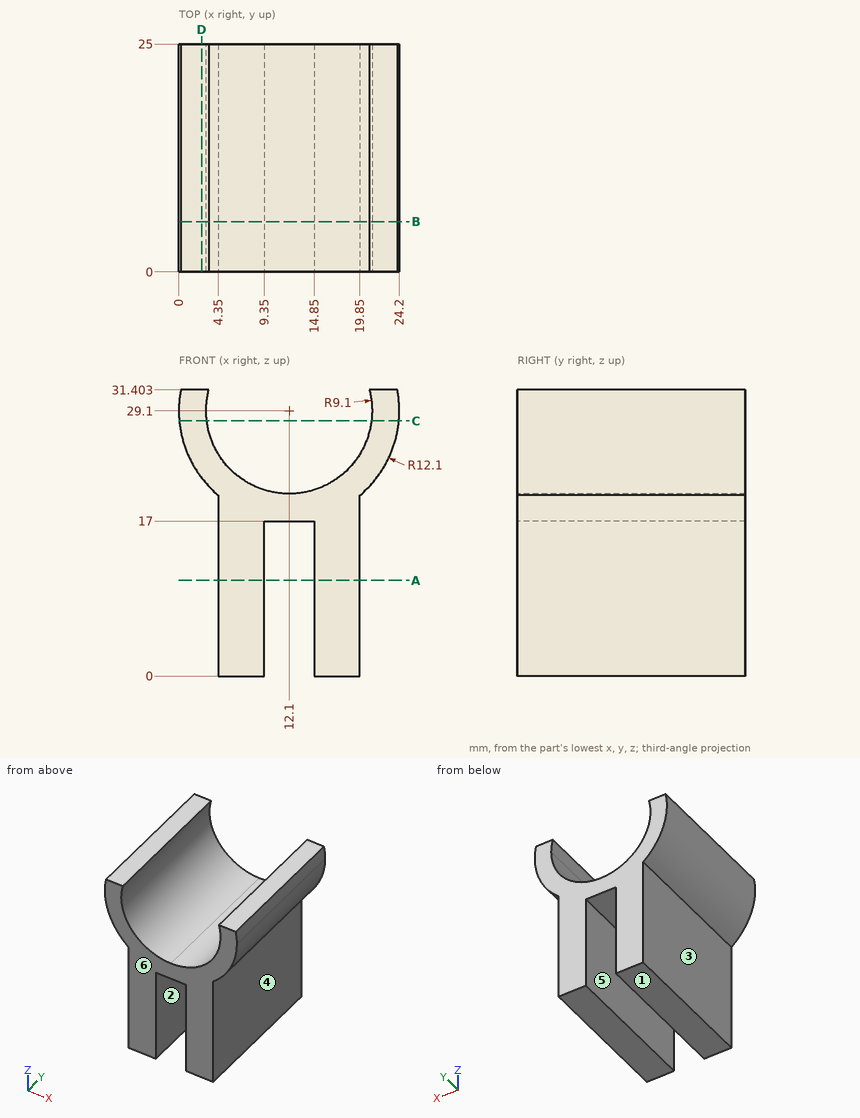
Answer from the drawing. Dimensions are ordinates in mm from the lowest x, y and z of the part. A direction names the side the tool comes from. Give positions to 0.01 mm unless a question says otherwise; leave off trailing zeros. Order: outer loops, then holes, each group sorted by start corner. A loop starts at its lowest first (then second) coordinate and runs counter-clockwise, first axis right, second up. Notation, with made-up numbers: (73.5, 29.25) - (131.5, 29.25) arc R21 cw to (131.5, 34.25) - close; hole circle Ø1 at (85.5, 7.25). An arc over 180 degrees is marked (long way). One line per item, written item: value. Start each with the question number.
1) Given pin 1 Ø3 at (x, y) = (12.5, 21.5) entering from -Z; pin 2 Ø12 at (y, z) = (6, 22.5) entering from -X (3 decimals); pin 3 Ø2 at (y, z) = (15, 20) entering from -X, each flat-ended and moving along its own axis, determine where each tip first touches the part or whether it passes through.
2) Find the intervals of material crossed by L1, parallel to X at y = 2.25, z = 6.5; L2, parallel to Z at x = 12, y = 15.25; L3, parallel to X at y = 21, z = 24, in increasing order.
3) The mould has two halves that part along X. Classify the marked faces 1, 2 and 3: released by +X, released by -X, zero draft, split by the parting line, or undercut.
4) A cutting plane is placed at C-C on z = 28. Give the vertices of the cut face in (x, y).
5) A cutting plane is placed at B-B on y = 5.5. Give the vertices of the cut face in (x, z), then the cut area to 3 significant figures.
6) A cutting plane is placed at D-D on x = 2.5. Give the vertices of the cut face in (y, z) (1 decimal), then the cut area to 3 significant figures.
7) A cutting plane is placed at A-A on z = 10.5. Give the vertices of the cut face in (x, y), then the cut area to 3 significant figures.
8) A tool of negligible diameter and unlimited length cuts with its end or side. For the marked faces 4, 5 and 6, from which of +Z, -Z, +X, -X, +Y, -Y can it reach the whole face along a straight path? Write none if from no direction.
Answer sheet:
1. pin 1: stops at z = 17
1. pin 2: stops at x = 0.015
1. pin 3: stops at x = 3.11
2. L1: x = 4.35 to 9.35, 14.85 to 19.85
2. L2: z = 17 to 20
2. L3: x = 1.13 to 4.56, 19.64 to 23.07
3. face 1: zero draft
3. face 2: undercut
3. face 3: released by -X
4. outline: (0.05, 0) - (3.07, 0) - (3.07, 25) - (0.05, 25) - close; (21.13, 0) - (24.15, 0) - (24.15, 25) - (21.13, 25) - close
5. outline: (0.22, 31.4) arc R12.1 ccw to (4.35, 19.81) - (4.35, 0) - (9.35, 0) - (9.35, 17) - (14.85, 17) - (14.85, 0) - (19.85, 0) - (19.85, 19.81) arc R12.1 ccw to (24.2, 29.1) arc R12.1 ccw to (23.98, 31.4) - (20.9, 31.4) arc R9.1 cw to (21.2, 29.1) arc R9.1 cw to (12.1, 20) arc R9.1 cw to (3.3, 31.4) - close
5. area: 298 mm2
6. outline: (0, 21.7) - (25, 21.7) - (25, 31.4) - (0, 31.4) - close
6. area: 242 mm2
7. outline: (4.35, 0) - (9.35, 0) - (9.35, 25) - (4.35, 25) - close; (14.85, 0) - (19.85, 0) - (19.85, 25) - (14.85, 25) - close
7. area: 250 mm2
8. face 4: -Z, +X, +Y, -Y
8. face 5: -Z, +Y, -Y
8. face 6: +Z, -Z, +X, -X, -Y
